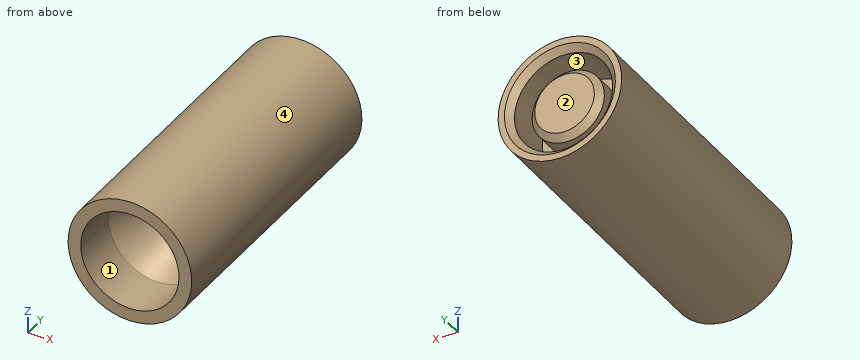
```python
from build123d import *

# Parameters (mm, degrees)
CHANFREIN1_SIZE = 0.4
CHANFREIN2_SIZE = 0.4


with BuildPart() as part:
    # Esquisse1 → Base-Révolution (revolve)
    with BuildSketch(Plane.XY, mode=Mode.PRIVATE) as base_r_volution_sk:
        with BuildLine():
            Line((-3.1, 0), (-3.9, 0))
            Line((-3.9, 0), (-3.9, 18.4))
            Line((-3.9, 18.4), (-3.1, 18.4))
            Line((-3.1, 18.4), (-3.1, 17.6))
            Line((-3.1, 17.6), (-3.1, 15))
            Line((-3.1, 15), (-2.279338742, 15))
            Line((-2.279338742, 15), (-2.279338742, 17.9))
            Line((-2.279338742, 17.9), (0, 17.9))
            Line((0, 17.9), (0, 16.9))
            Line((0, 16.9), (-1.5, 16.9))
            Line((-1.5, 16.9), (-1.5, 10.098076211))
            ThreePointArc((-1.5, 10.098076211), (-2.956912699, 8.006623421), (-2.279338742, 5.549457793))
            Line((-2.279338742, 5.549457793), (-3.1, 3))
            Line((-3.1, 3), (-3.1, 0.8))
            Line((-3.1, 0.8), (-3.1, 0))
        make_face()
    revolve(base_r_volution_sk.sketch.rotate(Axis((0, 0, 0), (0, 1, 0)), 270), axis=Axis((0, 0, 0), (0, 1, 0)))

    # Chanfrein1
    chanfrein1_edges = [part.edges().sort_by_distance(p)[0] for p in [
        (0, 18.4, 3.1),
    ]]
    chamfer(chanfrein1_edges, length=CHANFREIN1_SIZE)

    # Chanfrein2
    chanfrein2_edges = [part.edges().sort_by_distance(p)[0] for p in [
        (0, 17.9, 2.279338742),
    ]]
    chamfer(chanfrein2_edges, length=CHANFREIN2_SIZE)


solid = part.part
```
CAD build for the part. Positions are in the model's coordinates, mm. Face numbers are marked on the shaded views. A direction names the side the tool comes from. Round coordinates to 2 decimals unless told otherwise and drop trailing zeros. Loops run counter-clockwise (first coordinate to the right, second up) from the corner with the lowest first, then second, coordinate; pieces in that order, holes last. Notation, with made-up numbers: (-33.5, -10.75) - (-1.5, -10.75) arc R18 ccw to (-1.5, 22.25) - close; hole circle Ø2 at (36.25, -32). An arc over 180 degrees is marked (long way). Return JSON: item names as keys, results as strings. Group by question number.
Q1. Band-saw the part on A-A on z = 0. Give the cut face in (x, y).
Q2. Band-saw the part on C-C on y = 12.75. Give the cut face in (x, z).
Q3. Band-saw the part on D-D on y = 5. Give the cut face in (x, z).
Q4. Band-saw the part on B-B on x = 0. Give the cut face in (y, z).
Q5. Drill centre lines: line 1 along X through (y, z) = (15.9, 0); line 2 along X through (y, z) = (13.25, 0); line 3 along X through (y, z) = (15.75, 1.25). Where is each one in solid material? Low to high. Write a range as [from, to].
Q6. Two-plate mould, pull along Z, no slides. Class the marked faces 3 and 4: +Z half, -Z half, draft (parallel to the pull), parting line (faces both ways), or undercut.
Q7. Tool access for the marked faces 1 and 2: list every direction of +Z, -Z, +X, -X, +Y, -Y with a clear straight run to the whole face (end or side of a thin tool).
Q8. Flat gauge pins, fed straight in: pin 1 Ø1 at (x, y) = (-2, 11) entering from -Z; pin 2 Ø3 at (x, z) = (1.5, 1.5) entering from +Y; pin 3 Ø1.5 at (x, z) = (0.5, 0.5) entering from -Y; pin 4 Ø3.5 at (x, z) = (0, 0) entering from -Y. Where does each tip first touch, or does it go through?
Solutions:
{
 "1": {"outline": "(-3.9, 0) - (-3.1, 0) - (-3.1, 3) - (-2.28, 5.55) arc R3 cw to (-1.5, 10.1) - (-1.5, 16.9) - (1.5, 16.9) - (1.5, 10.1) arc R3 cw to (2.28, 5.55) - (3.1, 3) - (3.1, 0) - (3.9, 0) - (3.9, 18.4) - (3.5, 18.4) - (3.1, 18) - (3.1, 15) - (2.28, 15) - (2.28, 17.5) - (1.88, 17.9) - (-1.88, 17.9) - (-2.28, 17.5) - (-2.28, 15) - (-3.1, 15) - (-3.1, 18) - (-3.5, 18.4) - (-3.9, 18.4) - close"},
 "2": {"outline": "circle Ø7.8 at (0, 0); hole circle Ø3 at (0, 0)"},
 "3": {"outline": "circle Ø7.8 at (0, 0); hole circle Ø4.91 at (0, 0)"},
 "4": {"outline": "(0, -3.9) - (18.4, -3.9) - (18.4, -3.5) - (18, -3.1) - (15, -3.1) - (15, -2.28) - (17.5, -2.28) - (17.9, -1.88) - (17.9, 1.88) - (17.5, 2.28) - (15, 2.28) - (15, 3.1) - (18, 3.1) - (18.4, 3.5) - (18.4, 3.9) - (0, 3.9) - (0, 3.1) - (3, 3.1) - (5.55, 2.28) arc R3 cw to (10.1, 1.5) - (16.9, 1.5) - (16.9, -1.5) - (10.1, -1.5) arc R3 cw to (5.55, -2.28) - (3, -3.1) - (0, -3.1) - close"},
 "5": {"line 1": "x = [-3.9, -3.1], [-2.28, -1.5], [1.5, 2.28], [3.1, 3.9]", "line 2": "x = [-3.9, -1.5], [1.5, 3.9]", "line 3": "x = [-3.69, -2.84], [-1.91, -0.83], [0.83, 1.91], [2.84, 3.69]"},
 "6": {"face 3": "undercut", "face 4": "parting line"},
 "7": {"face 1": "-Y", "face 2": "+Y"},
 "8": {"pin 1": "stops at z = -3.6", "pin 2": "stops at y = 18.4", "pin 3": "stops at y = 16.9", "pin 4": "stops at y = 9.94"}
}
